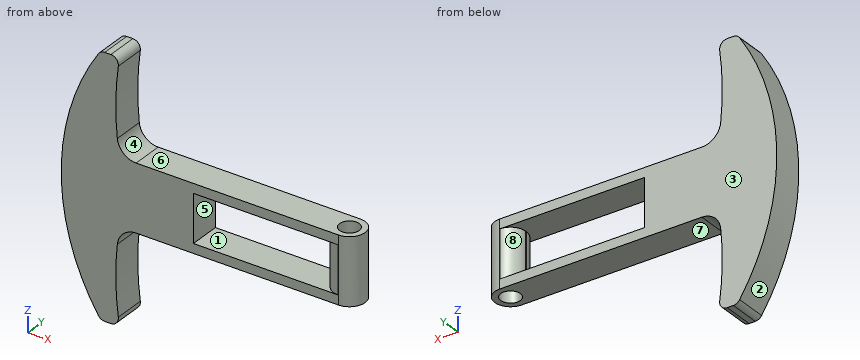
Autodesk Inventor part; units mm, degrees
ref_plane "YZ Plane" through (0, 0, 0) normal (1, 0, 0) x (0, 1, 0)
ref_plane "XZ Plane" through (0, 0, 0) normal (0, 1, 0) x (-1, 0, 0)
ref_plane "XY Plane" through (0, 0, 0) normal (0, 0, 1) x (1, 0, 0)
sketch "Sketch1" plane through (0, 0, 0) normal (0, 1, 0) x (-1, 0, 0)
  circle A0 centre (45.6085, 8.8) radius 5.405
  line L0 (3.774, 0.6) -> (39.2972, 0.6)
  line L1 (3.774, 17) -> (3.774, 0.6)
  line L2 (39.2972, 17) -> (3.774, 17)
  line L3 (39.2972, 0.6) -> (39.2972, 17)
  arc A1 (64.4148, -24.0966) -> (64.4148, 41.6966) centre (14.2369, 8.8) ccw
  line L4 (61.1267, 42.6) -> (62.7422, 42.6)
  line L5 (5.5105, 17.6) -> (54.4325, 17.6)
  line L6 (54.4325, 0) -> (5.5105, 0)
  line L7 (62.7422, -25) -> (61.1267, -25)
  line L8 (-3.1893, 17.6) -> (-3.1893, 0)
  line L9 (54.4325, 0) -> (-3.1893, 0)
  line L10 (-3.1893, 17.6) -> (58.8107, 17.6)
  arc A2 (59.144, -22.7375) -> (59.406, -4.4863) centre (-18.1812, -12.5) ccw
  arc A3 (59.406, 22.0863) -> (59.144, 40.3375) centre (-18.1812, 30.1) ccw
  arc A4 (59.406, -4.4863) -> (54.4325, 0) centre (54.4325, -5) ccw
  arc A5 (54.4325, 17.6) -> (59.406, 22.0863) centre (54.4325, 22.6) ccw
  arc A6 (62.7422, -25) -> (64.4148, -24.0966) centre (62.7422, -23) ccw
  arc A7 (59.144, -22.7375) -> (61.1267, -25) centre (61.1267, -23) ccw
  arc A8 (61.1267, 42.6) -> (59.144, 40.3375) centre (61.1267, 40.6) ccw
  arc A9 (64.4148, 41.6966) -> (62.7422, 42.6) centre (62.7422, 40.6) ccw
  point P0 (0, 0)
  point P1 (17.5306, 8.8)
  point P2 (63.8107, -25)
  point P3 (63.8107, 42.6)
  dimension "d0" = 17.6
  dimension "d1" = 62
  dimension "d2" = 78
  dimension "d3" = 78
  dimension "d4" = 5
  dimension "d5" = 2
extrude "Extrusion1" add sketch "Sketch1" along normal blind 8.3 contours A0 | L1 L2 L3 L0 | A6 L7 A7 A2 A4 L6 L9 L8 L10 L5 A5 A3 A8 L4 A9 A1
sketch "Sketch2" plane through (-54.4325, 0, 17.6) normal (0, 0, 1) x (1, 0, 0)
  line L0 (0, 0) -> (57.6218, 0) construction
  line L1 (57.6218, 0) -> (57.6218, 8.3)
  line L2 (0, 8.3) -> (57.6218, 8.3)
  line L3 (0, 0) -> (0, 8.3) construction
  line L4 (57.6218, 0) -> (57.6218, 8.3) construction
  line L5 (57.6218, 4.15) -> (52.9259, 4.15) construction
  circle A0 centre (53.4718, 4.15) radius 4.15
  circle A1 centre (53.4718, 4.15) radius 2.6
  line L6 (0, 8.3) -> (57.6218, 8.3)
  line L7 (57.6218, 0) -> (57.6218, 8.3) construction
  line L8 (0, 0) -> (57.6218, 0) construction
  line L9 (53.4718, 8.3) -> (57.6218, 8.3)
  line L10 (57.6218, 0) -> (57.6218, 8.3)
  line L11 (53.4718, 0) -> (57.6218, 0)
  point P0 (54.4325, 0)
  dimension "d8" = 1.55
extrude "Extrusion2" cut sketch "Sketch2" against normal through all
sketch "Sketch3" plane through (-54.4325, 0, 17.6) normal (0, 0, 1) x (1, 0, 0)
  circle A0 centre (53.4718, 4.15) radius 2.6 construction
  arc A1 (53.4718, 8.3) -> (53.4718, 0) centre (53.4718, 4.15) ccw construction
  circle A2 centre (53.4718, 4.15) radius 4.15
  point P0 (54.4325, 0)
extrude "Extrusion3" add sketch "Sketch3" against normal up to surface (17.6 mm away)
sketch "Sketch4" plane through (-54.4325, 0, 17.6) normal (0, 0, 1) x (1, 0, 0)
  circle A0 centre (53.4718, 4.15) radius 2.6
  point P0 (54.4325, 0)
extrude "Extrusion4" cut sketch "Sketch4" against normal through all
sketch "Sketch5" plane through (-54.4325, 0, 17.6) normal (0, 0, 1) x (1, 0, 0)
  point P0 (54.4325, 0)
sketch "Sketch6" plane through (0, 0, 0) normal (0, -1, 0) x (1, 0, 0)
  line L0 (-39.2972, 17) -> (-3.774, 17)
  line L1 (-39.2972, 0.6) -> (-39.2972, 17)
  line L2 (-3.774, 0.6) -> (-39.2972, 0.6)
  line L3 (-3.774, 17) -> (-3.774, 0.6)
  line L4 (-54.4325, 17.6) -> (-0.9607, 17.6) construction
  line L5 (-29.8249, 17.6) -> (-29.8249, 15.1) construction
  line L6 (-3.774, 14.6) -> (-3.774, 3)
  line L7 (-39.2972, 3) -> (-39.2972, 14.6)
  line L8 (-25.5022, 0) -> (-25.5022, 2.5)
  line L9 (-3.5607, 17.6) -> (-3.5607, 0) construction
  line L10 (-3.5607, 7.6434) -> (-5.0607, 7.6434) construction
  line L11 (-39.2972, 15.1) -> (-5.0607, 15.1)
  line L12 (-5.0607, 15.1) -> (-5.0607, 2.5)
  line L13 (-5.0607, 2.5) -> (-39.2972, 2.5)
  line L14 (-39.2972, 2.5) -> (-39.2972, 15.1)
  point P0 (0, 0)
  dimension "d15" = 2.5
  dimension "d16" = 11.6
  dimension "d19" = 2.5
  dimension "d20" = 1.5
extrude "Extrusion5" cut sketch "Sketch6" against normal blind 8.3 contours L11 L12 L13 L1
fillet "Fillet1" radius 4 2 edges at (-5.0607, 0, 8.8) (-5.0607, 8.3, 8.8)
properties part number "lever2"
Work out the finished part from the listing and answer in its coordinate system (mm). Face numbers are marked on the shaded views. A direction names the side the tool comes from. Give positions to 0.01 mm unless a question says otherwise; leave off trailing zeros. Loops run counter-clockwise (first coordinate to the right, second up) from the corner with the lowest first, then second, coordinate; pieces in that order, holes last. Notation, with made-up numbers: (-3.5, 9) -> (53.5, 9) arc R6 ccw to (53.5, 19) -> close; hole circle Ø9 at (-33, 42.5). An arc over 180 degrees is marked (long way). One line per question, with ' | ' between items. Start each with the question number.
1) Section A-A, the plane x = -20 is taken. Determine the outline of the cut face in (y, z).
2) Section C-C, the plane x = -52 is taken. Determine the outline of the cut face in (y, z).
3) Each of these flat-tipped pins is pushed along its axis until it touches: pin 1 (2 mm diameter, centred on x = -18.5, y = 4.5, fed in from +Z); pin 2 (4.5 mm diameter, centred on x = -0.96, y = 4.15, fed in from -Z); pin 3 (4 mm diameter, centred on x = -26, y = 6, fed in from -Z). Where does it stop, or does it pass through?
4) Section B-B, the plane z = 6 is taken. Determine the outline of the cut face in (x, y), then the cut area to 3 significant figures.
5) Straight lines are drawn through the part: L1, parallel to Z at x = -5, y = 7.5; L2, parallel to Z at x = -49, y = 6; L3, parallel to X at y = 2, z = 1.5. For each, find the intervals that lie inside material, in ascending order.
6) For the marked faces 5, 6, 7 and 8, determine the directions among +Z, -Z, +X, -X, +Y, -Y from which every point of the face is accessible in a straight line to the end or side of a thin tool.
7) Determine the mould class of the marked faces 1, 2, 3 and 4 for opening direction X: +X half, -X half, draft (parallel to the pull), parting line (faces both ways), or undercut.
Resolved:
1) outline: (0, 0) -> (8.3, 0) -> (8.3, 2.5) -> (0, 2.5) -> close; (0, 15.1) -> (8.3, 15.1) -> (8.3, 17.6) -> (0, 17.6) -> close
2) outline: (0, 0) -> (8.3, 0) -> (8.3, 17.6) -> (0, 17.6) -> close
3) pin 1: z = 17.6 | pin 2: through | pin 3: z = 0
4) outline: (-74.17, 0) -> (-39.3, 0) -> (-39.3, 8.3) -> (-74.17, 8.3) -> close; (-5.06, 4) arc R4 ccw to (-1.06, 0) -> (-0.96, 0) arc R4.15 ccw to (-0.96, 8.3) -> (-1.06, 8.3) arc R4 ccw to (-5.06, 4.3) -> close; hole circle Ø5.2 at (-0.96, 4.15) | area: 322 mm2
5) L1: 0 to 2.5, 15.1 to 17.6 | L2: 0 to 17.6 | L3: -73.79 to -2.42, 0.5 to 2.59
6) face 5: +Y, -Y | face 6: +Z, +X, +Y, -Y | face 7: -Z, +X, +Y, -Y | face 8: +Y
7) face 1: undercut | face 2: -X half | face 3: draft | face 4: +X half
